Work out the finished part from the listing and answer in its coordinate system (mm). A direction names the side the tool comes from. Coordinates: 2 decimals unless noted, no trailing zeros. Order: outer loops, then holes, each group sorted by start corner. A loop starts at its lowest first (then second) coordinate and runs counter-clockwise, first axis right, second up. Notation, with made-up numbers: M 43.5,-5 L 51.5,-5 A23 cw 51.5,16 Z; hole C 3,3.5 d4. An arc over 180 degrees is marked long. Use a Markdown table: item, result.
from build123d import *

# Parameters (mm, degrees)
ESBO_O1_W                = 130
ESBO_O1_H                = 50
RESSALTO_EXTRUS_O1_DEPTH = 15
ESBO_O2_W                = 110
ESBO_O2_H                = 10
CORTE_EXTRUS_O1_DEPTH    = 51
ESBO_O12_R               = 2
CORTE_EXTRUS_O8_DEPTH    = 10
CORTE_EXTRUS_O9_START    = -10
ESBO_O14_R               = 2
CORTE_EXTRUS_O9_DEPTH    = 10
ESBO_O7_R                = 2
CORTE_EXTRUS_O11_DEPTH   = 10
CORTE_EXTRUS_O12_START   = -10
ESBO_O6_R                = 2
CORTE_EXTRUS_O12_DEPTH   = 10
ESBO_O23_W               = 8.5
ESBO_O23_H               = 13
CORTE_EXTRUS_O13_DEPTH   = 10
ESBO_O20_W               = 30
ESBO_O20_H               = 3
CORTE_EXTRUS_O14_DEPTH   = 10


with BuildPart() as part:
    # Esboço1 → Ressalto-extrusão1 (new body)
    with BuildSketch(Plane(origin=(0, 0, 0), x_dir=(1, 0, 0), z_dir=(0, 1, 0))):
        with Locations((-65, 25)):
            Rectangle(ESBO_O1_W, ESBO_O1_H)
    extrude(amount=RESSALTO_EXTRUS_O1_DEPTH)

    # Esboço2 → Corte-extrusão1 (cut)
    with BuildSketch(Plane(origin=(0, 0, -50), x_dir=(-1, 0, 0), z_dir=(0, 0, -1))):
        with Locations((65, 5)):
            Rectangle(ESBO_O2_W, ESBO_O2_H)
    extrude(amount=-CORTE_EXTRUS_O1_DEPTH, mode=Mode.SUBTRACT)

    # Esboço12 → Corte-extrusão8 (cut)
    with BuildSketch(Plane(origin=(0, 0, 0), x_dir=(0, 0, -1), z_dir=(1, 0, 0))):
        with Locations((25, 5)):
            Circle(ESBO_O12_R)
    extrude(amount=-CORTE_EXTRUS_O8_DEPTH, mode=Mode.SUBTRACT)

    # Esboço14 → Corte-extrusão9 (cut)
    with BuildSketch(Plane.ZY.offset(130).offset(CORTE_EXTRUS_O9_START)):
        with Locations(Location((-25, 5, 0), (0, 0, 180))):
            Circle(ESBO_O14_R)
    extrude(amount=CORTE_EXTRUS_O9_DEPTH, mode=Mode.SUBTRACT)

    # Esboço7 → Corte-extrusão11 (cut)
    with BuildSketch(Plane.XY):
        with Locations((-5, 5)):
            Circle(ESBO_O7_R)
        with Locations((-125, 5)):
            Circle(ESBO_O7_R)
    extrude(amount=-CORTE_EXTRUS_O11_DEPTH, mode=Mode.SUBTRACT)

    # Esboço6 → Corte-extrusão12 (cut)
    with BuildSketch(Plane(origin=(0, 0, -50), x_dir=(-1, 0, 0), z_dir=(0, 0, -1)).offset(CORTE_EXTRUS_O12_START)):
        with Locations(Location((5, 5, 0), (0, 0, 180))):
            Circle(ESBO_O6_R)
        with Locations(Location((125, 5, 0), (0, 0, 180))):
            Circle(ESBO_O6_R)
    extrude(amount=CORTE_EXTRUS_O12_DEPTH, mode=Mode.SUBTRACT)

    # Esboço23 → Corte-extrusão13 (cut)
    with BuildSketch(Plane(origin=(0, 15, 0), x_dir=(1, 0, 0), z_dir=(0, 1, 0))):
        with Locations((-32.25, 25)):
            Rectangle(ESBO_O23_W, ESBO_O23_H)
    extrude(amount=-CORTE_EXTRUS_O13_DEPTH, mode=Mode.SUBTRACT)

    # Esboço20 → Corte-extrusão14 (cut)
    with BuildSketch(Plane(origin=(0, 15, 0), x_dir=(1, 0, 0), z_dir=(0, 1, 0))):
        with Locations((-95, 20.466517667)):
            Rectangle(ESBO_O20_W, ESBO_O20_H)
        with Locations((-95, 8.466517667)):
            Rectangle(ESBO_O20_W, ESBO_O20_H)
        with Locations((-95, 26.466517667)):
            Rectangle(ESBO_O20_W, ESBO_O20_H)
        with Locations((-95, 14.466517667)):
            Rectangle(ESBO_O20_W, ESBO_O20_H)
    extrude(amount=-CORTE_EXTRUS_O14_DEPTH, mode=Mode.SUBTRACT)


solid = part.part
(1) A cutting plane is placed at D-D (x = -116.5). Determine the outline of the cut face in (y, z).
Conclusion:
| item | result |
|---|---|
| outline | M 10,-50 L 15,-50 L 15,0 L 10,0 Z |
(2) A cutting plane is placed at B-B (x = -89). Determine the outline of the cut face in (y, z), then the cut area to 3 significant figures.
Conclusion:
| item | result |
|---|---|
| outline | M 10,-50 L 15,-50 L 15,-27.97 L 10,-27.97 Z; M 10,-24.97 L 15,-24.97 L 15,-21.97 L 10,-21.97 Z; M 10,-18.97 L 15,-18.97 L 15,-15.97 L 10,-15.97 Z; M 10,-12.97 L 15,-12.97 L 15,-9.97 L 10,-9.97 Z; M 10,-6.97 L 15,-6.97 L 15,0 L 10,0 Z |
| area | 190 mm2 |
(3) A cutting plane is placed at A-A (y = 11.5). Determine the outline of the cut face in (x, z).
Conclusion:
| item | result |
|---|---|
| outline | M -130,-50 L 0,-50 L 0,0 L -130,0 Z; hole M -110,-27.97 L -80,-27.97 L -80,-24.97 L -110,-24.97 Z; hole M -110,-21.97 L -80,-21.97 L -80,-18.97 L -110,-18.97 Z; hole M -110,-15.97 L -80,-15.97 L -80,-12.97 L -110,-12.97 Z; hole M -110,-9.97 L -80,-9.97 L -80,-6.97 L -110,-6.97 Z; hole M -36.5,-31.5 L -28,-31.5 L -28,-18.5 L -36.5,-18.5 Z |
(4) A cutting plane is placed at C-C (x = -5). Determine the outline of the cut face in (y, z).
Conclusion:
| item | result |
|---|---|
| outline | M 0,-50 L 3,-50 L 3,-40 L 7,-40 L 7,-50 L 15,-50 L 15,0 L 7,0 L 7,-10 L 3,-10 L 3,0 L 0,0 Z; hole C 5,-25 d4 |
(5) Determine the mould class of faces 1 (the flat face through (-125, 5, -40)), 2 (the flat face through (-130, 7.4, -24.7)), 3 (the cylindrical face through (-5, 5, -23)), 4 (the flat face through (-5, 5, -10)) for opening direction Z: pulls with the +Z half, pulls with the -Z half, needs draft (parallel to the pull), parting line crosses it, or undercut.
Conclusion:
| item | result |
|---|---|
| face 1 | pulls with the -Z half |
| face 2 | needs draft |
| face 3 | undercut |
| face 4 | pulls with the +Z half |
(6) Which of the six approach directions +Z, -Z, +X, -X, +Y, -Y give full straight-line access (tool end or side, diameter ignored) to faces 5 (the flat face through (-125, 5, -10)), 6 (the cylindrical face through (-127, 5, -45)), 7 (the flat face through (-110, 13, -20))?
Conclusion:
| item | result |
|---|---|
| face 5 | +Z |
| face 6 | -Z |
| face 7 | +Y, -Y |
(7) Straight lines are drawn through the part: L1, parallel to X at y = 5, z = -45; L2, parallel to Z at x = -125.75, y = 5; L3, parallel to Y at x = -125, z = -42.25. For each, find the intervals that lie inside material, in ascending order.
Conclusion:
| item | result |
|---|---|
| L1 | -130 to -127, -123 to -120, -10 to -7, -3 to 0 |
| L2 | -40 to -27, -23 to -10 |
| L3 | 0 to 3, 7 to 15 |
(8) Given P1, Ø2.5, axis at x = -91.5, y = 12, coming from the +Z side; P2, Ø10, axis at x = -24, z = -39, coming from the -Y side, each flat-ended and moving along its own axis, determine where each tip first touches the part or whether it passes through.
Conclusion:
| item | result |
|---|---|
| P1 | z = 0 |
| P2 | y = 10 |
